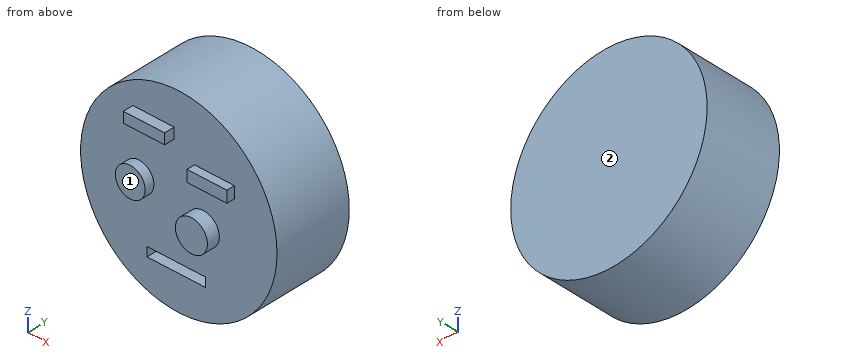
from build123d import *

# Parameters (mm, degrees)
F0_R        = 58.45034
F1_DEPTH    = 46.228
F2_W        = 24.600874
F2_H        = 6.29507
F3_DEPTH    = 6.096
F4_W        = 23.794292
F4_H        = 6.868821
F5_DEPTH    = 4.826
F6_R        = 8.879955
F7_DEPTH    = 5.588
F8_R        = 9.533495
F9_DEPTH    = 7.62
F1_FACE_R   = 58.45034
F1_FACE_R_2 = 8.879955
F1_FACE_R_3 = 9.533495
F1_FACE_W   = 24.600874
F1_FACE_H   = 6.29507
F1_FACE_W_2 = 23.794292
F1_FACE_H_2 = 6.86882
F11_DEPTH   = 6.604
F12_W       = 34.83605
F12_H       = 5.481868
F13_DEPTH   = 11.176


with BuildPart() as f1:
    # F0 (on Front) → F1 (new body)
    with BuildSketch(Plane.XZ):
        with Locations((-49.329195, 18.883251)):
            Circle(F0_R)
    extrude(amount=F1_DEPTH)

    # F2 (on face) → F3 (join)
    with BuildSketch(Plane.XZ.offset(46.228)):
        with Locations((-64.380275, 53.784102)):
            Rectangle(F2_W, F2_H)
    extrude(amount=F3_DEPTH)

    # F4 (on face) → F5 (join)
    with BuildSketch(Plane.XZ.offset(46.228)):
        with Locations((-28.083899, 39.257792)):
            Rectangle(F4_W, F4_H)
    extrude(amount=F5_DEPTH)

    # F6 (on face) → F7 (join)
    with BuildSketch(Plane.XZ.offset(46.228)):
        with Locations((-73.05108, 21.034079)):
            Circle(F6_R)
    extrude(amount=F7_DEPTH)

    # F8 (on face) → F9 (join)
    with BuildSketch(Plane.XZ.offset(46.228)):
        with Locations((-34.738239, 11.52609)):
            Circle(F8_R)
    extrude(amount=F9_DEPTH)

    # F1_face (on face) → F11 (join)
    with BuildSketch(Plane(origin=(-49.329195, -46.228, 18.883251), x_dir=(1, 0, 0), z_dir=(0, -1, 0))):
        Circle(F1_FACE_R)
        with Locations((-23.721885, 2.150828)):
            Circle(F1_FACE_R_2, mode=Mode.SUBTRACT)
        with Locations((14.590956, -7.357161)):
            Circle(F1_FACE_R_3, mode=Mode.SUBTRACT)
        with Locations((-15.05108, 34.900852)):
            Rectangle(F1_FACE_W, F1_FACE_H, mode=Mode.SUBTRACT)
        with Locations((21.245296, 20.374542)):
            Rectangle(F1_FACE_W_2, F1_FACE_H_2, mode=Mode.SUBTRACT)
    extrude(amount=-F11_DEPTH)

    # F12 (on face) → F13 (cut)
    with BuildSketch(Plane.XZ.offset(46.228)):
        with Locations((-50.854826, -16.175416)):
            Rectangle(F12_W, F12_H)
    extrude(amount=-F13_DEPTH, mode=Mode.SUBTRACT)


solid = f1.part
Input: part model. Units: mm. Frame: model coordinates. Face numbers are marked on the shaded views. A direction names the side the tool comes from. Round coordinates to 2 decimals unless told otherwise and drop trailing zeros. Write each loop counter-clockwise with the first axis right and the second up, starting at its lowest first coordinate (ties: lowest second). Pieces come first, ordered by that corner, then holes.
1) Cut plane D-D (z = 52.5). Return the cut outline in (x, y).
2) Cut plane B-B (z = 5.5). Return the cut outline in (x, y), then the cut area to 3 significant figures.
3) Contact query for flat-ended pins moving along their axis: P1, Ø3.5, axis at x = -57, y = -39.5, coming from the +Z side; P2, Ø2, axis at x = -54.5, y = -43.5, coming from the -Z side; P3, Ø3, axis at x = -61.5, y = -50, coming from the -Z side; P4, Ø4, axis at x = -60, z = 57, coming from the +Y side. Output: stop coordinate, or through.
4) Cut plane C-C (y = -37.5). Return the cut outline in (x, z).
5) Ray query, L1, parallel to Z at x = -50, y = -43.5; L2, parallel to Y at x = -44, z = -5.5; L3, parallel to Z at x = -51, y = -12.5. Return the intervals inside material, ascending.
6) Cut plane A-A (x = -35). Return the cut outline in (y, z).
7) Reachability of the marked faces 1 and 2 from +Z, -Z, +X, -X, +Y, -Y: full face, straight path, thin tool, end or side. Return the list, or none.
Geometry says:
1. outline: (-97.15, -46.23) - (-76.68, -46.23) - (-76.68, -52.32) - (-52.08, -52.32) - (-52.08, -46.23) - (-1.51, -46.23) - (-1.51, 0) - (-97.15, 0) - close
2. outline: (-106.23, -46.23) - (-42.13, -46.23) - (-42.13, -53.85) - (-27.35, -53.85) - (-27.35, -46.23) - (7.57, -46.23) - (7.57, 0) - (-106.23, 0) - close
2. area: 5,370 mm2
3. P1: stops at z = 77.03
3. P2: stops at z = -39.42
3. P3: stops at z = 50.64
3. P4: stops at y = 0
4. outline: circle Ø116.9 at (-49.33, 18.88); hole (-68.27, -18.92) - (-33.44, -18.92) - (-33.44, -13.43) - (-68.27, -13.43) - close
5. L1: z = -39.56 to -18.92, -13.43 to 77.33
5. L2: y = -46.23 to 0
5. L3: z = -39.54 to 77.31
6. outline: (-53.85, 2) - (-46.23, 2) - (-46.23, -13.43) - (-35.05, -13.43) - (-35.05, -18.92) - (-46.23, -18.92) - (-46.23, -37.78) - (0, -37.78) - (0, 75.55) - (-46.23, 75.55) - (-46.23, 42.69) - (-51.05, 42.69) - (-51.05, 35.82) - (-46.23, 35.82) - (-46.23, 21.06) - (-53.85, 21.06) - close
7. face 1: -Z, -X, -Y
7. face 2: +Z, -Z, +X, -X, +Y
